```python
from build123d import *

# Parameters (mm, degrees)
SKETCH1_W                      = 25.4
SKETCH1_H                      = 25.4
SKETCH1_W_2                    = 19.812
SKETCH1_H_2                    = 19.812
BOSS_EXTRUDE1_DEPTH            = 25.4
SKETCH4_W                      = 25.4
SKETCH4_H                      = 25.4
BOSS_EXTRUDE2_DEPTH            = 6.35
F_6_CLEARANCE_HOLE2_D          = 3.7973
F_6_CLEARANCE_HOLE2_DEPTH      = 9.144
CUT_EXTRUDE1_DEPTH             = 5.08
CUT_EXTRUDE1_DIRECTION_2_REACH = 38.297
SKETCH8_W                      = 25.4
SKETCH8_H                      = 9.905999957
BOSS_EXTRUDE4_DEPTH            = 1.4224
SKETCH9_W                      = 25.4
SKETCH9_H                      = 25.4
BOSS_EXTRUDE5_DEPTH            = 6.35
CUT_EXTRUDE2_REACH             = 46.45
SKETCH10_R                     = 6.5
M3_CLEARANCE_HOLE1_D           = 3.4
CIRPATTERN1_COUNT              = 4
FILLET1_R                      = 12.7
SKETCH15_W                     = 19.812
SKETCH15_H                     = 19.812
SKETCH15_W_2                   = 16.002
SKETCH15_H_2                   = 16.002
BOSS_EXTRUDE6_DEPTH            = 2.54
SKETCH17_R                     = 3.25
CUT_EXTRUDE4_DEPTH             = 2.75
CIRPATTERN2_COUNT              = 4
FILLET4_R                      = 1.27
F_4_CLEARANCE_HOLE1_D          = 3.2639
CHAMFER1_SIZE                  = 1.4224
CHAMFER2_SIZE                  = 1.27
SKETCH22_W                     = 10.16
SKETCH22_H                     = 2.54
BOSS_EXTRUDE7_DEPTH            = 5.08
CHAMFER3_SIZE                  = 2.54
BOSS_EXTRUDE8_DEPTH            = 5.08
BOSS_EXTRUDE9_DEPTH            = 2.153
BOSS_EXTRUDE10_DEPTH           = 3.677


with BuildPart() as part:
    # Sketch1 → Boss-Extrude1 (new body)
    with BuildSketch(Plane(origin=(0, 0, 0), x_dir=(1, 0, 0), z_dir=(0, 1, 0))):
        Rectangle(SKETCH1_W, SKETCH1_H)
        Rectangle(SKETCH1_W_2, SKETCH1_H_2, mode=Mode.SUBTRACT)
    extrude(amount=BOSS_EXTRUDE1_DEPTH)

    # Sketch4 → Boss-Extrude2 (add)
    with BuildSketch(Plane(origin=(12.7, 0, 0), x_dir=(0, 0, -1), z_dir=(1, 0, 0))):
        with Locations((0, 12.7)):
            Rectangle(SKETCH4_W, SKETCH4_H)
    extrude(amount=BOSS_EXTRUDE2_DEPTH)

    # #6 Clearance Hole2
    with Locations(Plane(origin=(19.05, 0, 0), x_dir=(0, 0, -1), z_dir=(1, 0, 0))):
        with Locations((5.588, 8.128000043)):
            Hole(F_6_CLEARANCE_HOLE2_D / 2, depth=F_6_CLEARANCE_HOLE2_DEPTH)

    # Sketch7 → Cut-Extrude1 (cut)
    with BuildSketch(Plane.ZY.offset(-9.906)):
        Polygon((-5.588, 13.260643936), (-10.033, 10.69432199), (-10.033, 5.561678096), (-5.588, 2.99535615), (-1.143, 5.561678096), (-1.143, 10.69432199), align=None)
    extrude(amount=-CUT_EXTRUDE1_DEPTH, mode=Mode.SUBTRACT)

    # Cut-Extrude1 direction 2: up to this face of the body (flat: up to its plane)
    cut_extrude1_direction_2_end = Plane(part.part.faces().sort_by_distance((-9.906, 12.7, 0))[0])
    # Sketch7 → Cut-Extrude1 direction 2 (cut, up to the picked face)
    with BuildSketch(Plane.ZY.offset(-9.906), mode=Mode.PRIVATE) as cut_extrude1_direction_2_sk1:
        Polygon((-5.588, 13.260643936), (-10.033, 10.69432199), (-10.033, 5.561678096), (-5.588, 2.99535615), (-1.143, 5.561678096), (-1.143, 10.69432199), align=None)
    cut_extrude1_direction_2_tool1 = split(extrude(cut_extrude1_direction_2_sk1.sketch, amount=CUT_EXTRUDE1_DIRECTION_2_REACH, mode=Mode.PRIVATE), bisect_by=cut_extrude1_direction_2_end, keep=Keep.BOTH, mode=Mode.PRIVATE)
    add(cut_extrude1_direction_2_tool1.solids().sort_by(Axis((9.906, 8.128, -5.588), (-1, 0, 0)))[0], mode=Mode.SUBTRACT)

    # Sketch8 → Boss-Extrude4 (add)
    with BuildSketch(Plane(origin=(19.05, 0, 0), x_dir=(0, 0, -1), z_dir=(1, 0, 0))):
        with Locations((0, 20.447000022)):
            Rectangle(SKETCH8_W, SKETCH8_H)
    extrude(amount=BOSS_EXTRUDE4_DEPTH)

    # Sketch9 → Boss-Extrude5 (add)
    with BuildSketch(Plane.XZ):
        with Locations((-25.4, 0)):
            Rectangle(SKETCH9_W, SKETCH9_H)
    extrude(amount=-BOSS_EXTRUDE5_DEPTH)

    # Sketch10 → Cut-Extrude2 (cut, up to next)
    with BuildSketch(Plane(origin=(0, 6.35, 0), x_dir=(1, 0, 0), z_dir=(0, 1, 0)), mode=Mode.PRIVATE) as cut_extrude2_sk1:
        with Locations(Location((-25.4, 0, 0), (0, 0, 270))):
            Circle(SKETCH10_R)
    cut_extrude2_tool1 = extrude(cut_extrude2_sk1.sketch, amount=-CUT_EXTRUDE2_REACH, mode=Mode.PRIVATE) & part.part
    add(cut_extrude2_tool1.solids().sort_by_distance((-25.4, 6.35, 0))[0], mode=Mode.SUBTRACT)

    # M3 Clearance Hole1 (through all)
    with Locations(Plane(origin=(0, 6.35, 0), x_dir=(1, 0, 0), z_dir=(0, 1, 0))):
        with Locations((-25.4, 9)):
            m3_clearance_hole1 = Hole(M3_CLEARANCE_HOLE1_D / 2)

    # CirPattern1: M3 Clearance Hole1 ×4 about axis
    cirpattern1_axis = Axis((-25.4, 0, 0), (0, 1, 0))
    for i in range(1, CIRPATTERN1_COUNT):
        add(m3_clearance_hole1.rotate(cirpattern1_axis, i * 360 / CIRPATTERN1_COUNT), mode=Mode.SUBTRACT)

    # Fillet1
    fillet1_edges = [part.edges().sort_by_distance(p)[0] for p in [
        (-38.1, 3.175, 12.7),
        (-38.1, 3.175, -12.7),
    ]]
    fillet(fillet1_edges, radius=FILLET1_R - 0.0001)  # a hair under: the kernel refuses the full size

    # Sketch15 → Boss-Extrude6 (add)
    with BuildSketch(Plane.XZ):
        Rectangle(SKETCH15_W, SKETCH15_H)
        Rectangle(SKETCH15_W_2, SKETCH15_H_2, mode=Mode.SUBTRACT)
    extrude(amount=-BOSS_EXTRUDE6_DEPTH)

    # Sketch17 → Cut-Extrude4 (cut)
    with BuildSketch(Plane(origin=(0, 6.35, 0), x_dir=(1, 0, 0), z_dir=(0, 1, 0))):
        with Locations((-25.4, 9)):
            Circle(SKETCH17_R)
    cut_extrude4 = extrude(amount=-CUT_EXTRUDE4_DEPTH, mode=Mode.SUBTRACT)

    # CirPattern2: Cut-Extrude4 ×4 about axis
    cirpattern2_axis = Axis((-25.4, 0, 0), (0, 1, 0))
    for i in range(1, CIRPATTERN2_COUNT):
        add(cut_extrude4.rotate(cirpattern2_axis, i * 360 / CIRPATTERN2_COUNT), mode=Mode.SUBTRACT)

    # Fillet4
    fillet4_edges = [part.edges().sort_by_distance(p)[0] for p in [
        (-8.001, 2.54, 0),
        (0, 2.54, -8.001),
        (8.001, 2.54, 0),
        (0, 2.54, 8.001),
        (-8.001, 0, 0),
        (-8.001, 1.27, 8.001),
        (0, 0, 8.001),
        (8.001, 1.27, 8.001),
        (8.001, 0, 0),
        (8.001, 1.27, -8.001),
        (0, 0, -8.001),
        (-8.001, 1.27, -8.001),
    ]]
    fillet(fillet4_edges, radius=FILLET4_R - 0.0001)  # a hair under: the kernel refuses the full size

    # #4 Clearance Hole1 (through all)
    with Locations(Plane(origin=(0, 0, -12.7), x_dir=(-1, 0, 0), z_dir=(0, 0, -1))):
        with Locations((0, 6.35)):
            Hole(F_4_CLEARANCE_HOLE1_D / 2)

    # Chamfer1
    chamfer1_edges = [part.edges().sort_by_distance(p)[0] for p in [
        (20.4724, 15.494000043, 0),
    ]]
    chamfer(chamfer1_edges, length=CHAMFER1_SIZE - 0.0001)  # a hair under: the kernel refuses the full size

    # Chamfer2
    chamfer2_edges = [part.edges().sort_by_distance(p)[0] for p in [
        (9.906, 25.4, 0),
        (0, 25.4, -9.906),
        (-9.906, 25.4, 0),
        (0, 25.4, 9.906),
    ]]
    chamfer(chamfer2_edges, length=CHAMFER2_SIZE)

    # Sketch22 → Boss-Extrude7 (add)
    with BuildSketch(Plane(origin=(0, 0, -12.7), x_dir=(-1, 0, 0), z_dir=(0, 0, -1))):
        with Locations((2.54, 1.27)):
            Rectangle(SKETCH22_W, SKETCH22_H)
    extrude(amount=BOSS_EXTRUDE7_DEPTH)

    # Chamfer3
    chamfer3_edges = [part.edges().sort_by_distance(p)[0] for p in [
        (-7.62, 1.27, -17.78),
        (2.54, 1.27, -17.78),
    ]]
    chamfer(chamfer3_edges, length=CHAMFER3_SIZE)

    # Sketch23 → Boss-Extrude8 (add)
    with BuildSketch(Plane(origin=(0, 0, -12.7), x_dir=(-1, 0, 0), z_dir=(0, 0, -1))):
        Polygon((12.7, 9.999), (12.7, 22.16), (10.547, 22.16), (10.547, 12.152), (9.023, 12.152), (9.023, 9.999), align=None)
        Polygon((-7.487, 25.4), (-12.18, 25.4), (-12.18, 12.66), (-10.027, 12.66), (-10.027, 23.368), (-7.487, 23.368), align=None)
    extrude(amount=BOSS_EXTRUDE8_DEPTH)

    # Sketch24 → Boss-Extrude9 (add)
    with BuildSketch(Plane(origin=(12.18, 0, 0), x_dir=(0, 0, -1), z_dir=(1, 0, 0))):
        Polygon((17.78, 12.66), (12.7, 12.66), (12.7, 7.58), align=None)
    extrude(amount=-BOSS_EXTRUDE9_DEPTH)

    # Sketch25 → Boss-Extrude10 (add)
    with BuildSketch(Plane.ZY.offset(12.7)):
        Polygon((-17.78, 9.999), (-12.7, 9.999), (-12.7, 4.919), align=None)
    extrude(amount=-BOSS_EXTRUDE10_DEPTH)


solid = part.part
```
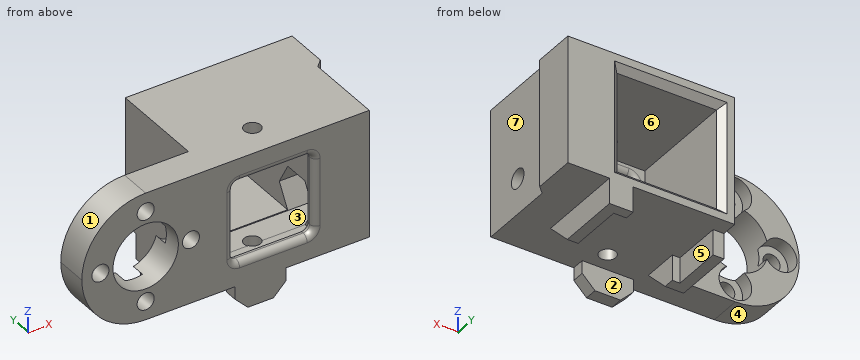
CAD build for the part. Positions are in the model's coordinates, mm. Face numbers are marked on the shaded views. A direction names the side the tool comes from. Round coordinates to 2 decimals unless told otherwise and drop trailing zeros. Loops run counter-clockwise (first coordinate to the right, second up) from the corner with the lowest first, then second, coordinate; pieces in that order, holes last. Notation, with made-up numbers: (45.5, -5.75) - (80.5, -5.75) arc R31 cw to (80.5, 22.25) - close; hole circle Ø11 at (77, -39.5). An arc over 180 degrees is marked (long way). Return JSON: item names as keys, results as strings. Group by question number.
Q1. Two-plate mould, pull along Z, no slides. Class the marked faces 1, 2, 3 and 4: +Z half, -Z half, draft (parallel to the pull), parting line (faces both ways), or undercut.
Q2. Band-saw the part on B-B on y = 14. Give the cut face in (x, z), plus the area to 3 significant figures.
Q3. Flat gauge pins, fed straight in: pin 1 Ø10 at (y, z) = (6.5, -5.5) entering from -X; pin 2 Ø3 at (x, z) = (-17, -1) entering from +Y; pin 3 Ø4 at (y, z) = (18, -12.5) entering from -X. Where does each tip first touch, or does it go through?
Q4. Drill centre lines: line 1 along X through (y, z) = (2.9, 0); line 2 along Z through (x, y) = (-16.4, 5.75); line 3 along X through (y, z) = (18.75, 9). Where is each one in solid material? Low to high. Write a range as [from, to].
Q5. Band-saw the part on A-A on x = -16.4. Give the cut face in (y, z), plus the area to 3 significant figures.
Q6. Band-saw the part on D-D on x = -34.4. Give the cut face in (y, z), plus the area to 3 significant figures.
Q7. Tool access for the marked faces 5, 6 and 7: list every direction of +Z, -Z, +X, -X, +Y, -Y with a clear straight run to the whole face (end or side of a thin tool).
Solutions:
{
 "1": {"face 1": "+Z half", "face 2": "draft", "face 3": "undercut", "face 4": "-Z half"},
 "2": {"outline": "(-12.7, -17.78) - (-10.55, -17.78) - (-10.55, -12.7) - (10.03, -12.7) - (10.03, -17.78) - (12.18, -17.78) - (12.18, -12.7) - (19.05, -12.7) - (19.05, 12.7) - (-12.7, 12.7) - close; hole (-9.91, -9.91) - (9.91, -9.91) - (9.91, 9.91) - (-9.91, 9.91) - close", "area": "436 mm^2"},
 "3": {"pin 1": "stops at x = -38.09", "pin 2": "stops at y = 3.6", "pin 3": "stops at x = -12.7"},
 "4": {"line 1": "x = [-38.1, -36.1], [-32.7, -31.9], [-18.9, -18.1], [-14.7, -9.91], [9.91, 19.05]", "line 2": "z = [-12.7, -3.25], [3.25, 12.7]", "line 3": "x = [-12.7, -9.91], [9.91, 20.47]"},
 "5": {"outline": "(0, -12.7) - (6.35, -12.7) - (6.35, -3.25) - (3.6, -3.25) - (3.6, -1.7) - (0, -1.7) - close; (0, 1.7) - (3.6, 1.7) - (3.6, 3.25) - (6.35, 3.25) - (6.35, 12.7) - (0, 12.7) - close", "area": "131 mm^2"},
 "6": {"outline": "(0, -8.96) - (6.35, -8.96) - (6.35, -3.25) - (3.6, -3.25) - (3.6, -1.7) - (0, -1.7) - close; (0, 1.7) - (3.6, 1.7) - (3.6, 3.25) - (6.35, 3.25) - (6.35, 8.96) - (0, 8.96) - close", "area": "83.7 mm^2"},
 "7": {"face 5": "-Z, +Y", "face 6": "+Y", "face 7": "+Z, -Z, +X, -Y"}
}
